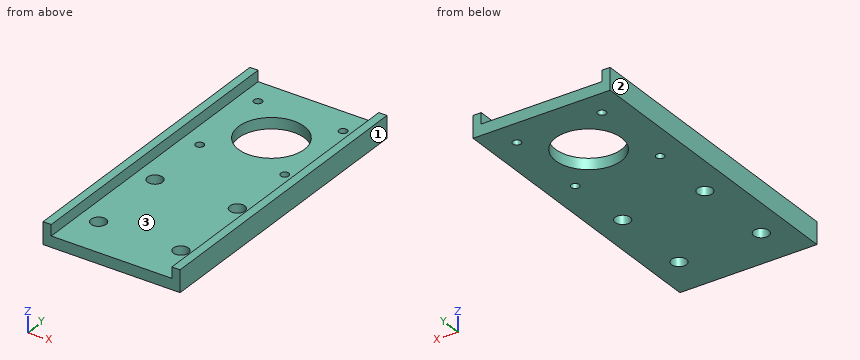
```python
from build123d import *

# Parameters (mm, degrees)
SKETCH1_W           = 50
SKETCH1_H           = 110
BOSS_EXTRUDE1_DEPTH = 4
CUT_EXTRUDE1_REACH  = 62.548
SKETCH2_R           = 1.5
CUT_EXTRUDE2_REACH  = 62.548
SKETCH3_R           = 2.75
SKETCH4_W           = 3
SKETCH4_H           = 110
BOSS_EXTRUDE2_DEPTH = 8
CUT_EXTRUDE3_REACH  = 62.943
SKETCH5_R           = 12


with BuildPart() as part:
    # Sketch1 → Boss-Extrude1 (new body)
    with BuildSketch(Plane.XY):
        Rectangle(SKETCH1_W, SKETCH1_H)
    extrude(amount=BOSS_EXTRUDE1_DEPTH)

    # Sketch2 → Cut-Extrude1 (cut, up to next)
    with BuildSketch(Plane.XY, mode=Mode.PRIVATE) as cut_extrude1_sk1:
        with Locations((-15.5, 45.5)):
            Circle(SKETCH2_R)
    cut_extrude1_tool1 = extrude(cut_extrude1_sk1.sketch, amount=CUT_EXTRUDE1_REACH, mode=Mode.PRIVATE) & part.part
    # Sketch2 → Cut-Extrude1 (cut, up to next)
    with BuildSketch(Plane.XY, mode=Mode.PRIVATE) as cut_extrude1_sk2:
        with Locations((-15.5, 14.5)):
            Circle(SKETCH2_R)
    cut_extrude1_tool2 = extrude(cut_extrude1_sk2.sketch, amount=CUT_EXTRUDE1_REACH, mode=Mode.PRIVATE) & part.part
    # Sketch2 → Cut-Extrude1 (cut, up to next)
    with BuildSketch(Plane.XY, mode=Mode.PRIVATE) as cut_extrude1_sk3:
        with Locations(Location((15.5, 14.5, 0), (0, 0, 180))):
            Circle(SKETCH2_R)
    cut_extrude1_tool3 = extrude(cut_extrude1_sk3.sketch, amount=CUT_EXTRUDE1_REACH, mode=Mode.PRIVATE) & part.part
    # Sketch2 → Cut-Extrude1 (cut, up to next)
    with BuildSketch(Plane.XY, mode=Mode.PRIVATE) as cut_extrude1_sk4:
        with Locations(Location((15.5, 45.5, 0), (0, 0, 180))):
            Circle(SKETCH2_R)
    cut_extrude1_tool4 = extrude(cut_extrude1_sk4.sketch, amount=CUT_EXTRUDE1_REACH, mode=Mode.PRIVATE) & part.part
    add(cut_extrude1_tool1.solids().sort_by_distance((-15.5, 45.5, 0))[0], mode=Mode.SUBTRACT)
    add(cut_extrude1_tool2.solids().sort_by_distance((-15.5, 14.5, 0))[0], mode=Mode.SUBTRACT)
    add(cut_extrude1_tool3.solids().sort_by_distance((15.5, 14.5, 0))[0], mode=Mode.SUBTRACT)
    add(cut_extrude1_tool4.solids().sort_by_distance((15.5, 45.5, 0))[0], mode=Mode.SUBTRACT)

    # Sketch3 → Cut-Extrude2 (cut, up to next)
    with BuildSketch(Plane.XY, mode=Mode.PRIVATE) as cut_extrude2_sk1:
        with Locations((-15, -40)):
            Circle(SKETCH3_R)
    cut_extrude2_tool1 = extrude(cut_extrude2_sk1.sketch, amount=CUT_EXTRUDE2_REACH, mode=Mode.PRIVATE) & part.part
    # Sketch3 → Cut-Extrude2 (cut, up to next)
    with BuildSketch(Plane.XY, mode=Mode.PRIVATE) as cut_extrude2_sk2:
        with Locations((-15, -10)):
            Circle(SKETCH3_R)
    cut_extrude2_tool2 = extrude(cut_extrude2_sk2.sketch, amount=CUT_EXTRUDE2_REACH, mode=Mode.PRIVATE) & part.part
    # Sketch3 → Cut-Extrude2 (cut, up to next)
    with BuildSketch(Plane.XY, mode=Mode.PRIVATE) as cut_extrude2_sk3:
        with Locations(Location((15, -40, 0), (0, 0, 180))):
            Circle(SKETCH3_R)
    cut_extrude2_tool3 = extrude(cut_extrude2_sk3.sketch, amount=CUT_EXTRUDE2_REACH, mode=Mode.PRIVATE) & part.part
    # Sketch3 → Cut-Extrude2 (cut, up to next)
    with BuildSketch(Plane.XY, mode=Mode.PRIVATE) as cut_extrude2_sk4:
        with Locations(Location((15, -10, 0), (0, 0, 180))):
            Circle(SKETCH3_R)
    cut_extrude2_tool4 = extrude(cut_extrude2_sk4.sketch, amount=CUT_EXTRUDE2_REACH, mode=Mode.PRIVATE) & part.part
    add(cut_extrude2_tool1.solids().sort_by_distance((-15, -40, 0))[0], mode=Mode.SUBTRACT)
    add(cut_extrude2_tool2.solids().sort_by_distance((-15, -10, 0))[0], mode=Mode.SUBTRACT)
    add(cut_extrude2_tool3.solids().sort_by_distance((15, -40, 0))[0], mode=Mode.SUBTRACT)
    add(cut_extrude2_tool4.solids().sort_by_distance((15, -10, 0))[0], mode=Mode.SUBTRACT)

    # Sketch4 → Boss-Extrude2 (add)
    with BuildSketch(Plane.XY):
        with Locations((-23.5, 0)):
            Rectangle(SKETCH4_W, SKETCH4_H)
        with Locations((23.5, 0)):
            Rectangle(SKETCH4_W, SKETCH4_H)
    extrude(amount=BOSS_EXTRUDE2_DEPTH)

    # Sketch5 → Cut-Extrude3 (cut, up to next)
    with BuildSketch(Plane.XY, mode=Mode.PRIVATE) as cut_extrude3_sk1:
        with Locations((0, 30)):
            Circle(SKETCH5_R)
    cut_extrude3_tool1 = extrude(cut_extrude3_sk1.sketch, amount=CUT_EXTRUDE3_REACH, mode=Mode.PRIVATE) & part.part
    add(cut_extrude3_tool1.solids().sort_by_distance((0, 30, 0))[0], mode=Mode.SUBTRACT)


solid = part.part
```
Design review of the part built by this model. Coordinates are the model's own, in mm. Face numbers are marked on the shaded views. Round coordinates to 2 decimals unless told otherwise and drop trailing zeros. Write each loop counter-clockwise with the first axis right and the second up, starting at its lowest first coordinate (ties: lowest second). Pieces come first, ordered by that corner, then holes. Notation, with made-up numbers: (25, -34) -> (58, -34) arc R30 ccw to (58, -1) -> close; hole circle Ø1 at (-24, 35). An arc over 180 degrees is marked (long way). Write item = value, one per line. Start each with the question number.
1) Wall thickness on probe 1 along X at (y, z) = (-10, 1.05); probe 2 along X at (y, z) = (45.5, 1.3); probe 3 along Y at (x, z) = (15.5, 1.1): over which ranges is each line inside the solid? List them lowest first. Write a range as from..to.
2) Take a section at D-D, the plane z = 1. Count the separate pieces of the cut face and the enclosed holes in it, plus the area to 3 significant figures.
3) Take a section at B-B, the plane z = 6.75. State the section outline as (x, y) points, plus the area to 3 significant figures.
4) Mouldability with a two-part tool opening along X and no side actions: class the marked faces 1, 2 and 3 as +X half, -X half, draft (parallel to the pull), parting line (faces both ways), or undercut.
5) Take a section at C-C, the plane y = 30. State the section outline as (x, z) points.
6) Take a section at A-A, the plane x = 0. State the section outline as (y, z) points.
7) Clearance check with a flat-ended pin moving along its axis: pin 1 (10 mm diameter, centred on x = 2.5, y = 39.5, fed in from +Z). State where the tip first meets the part, or that it passes through.
Results list:
q1.probe_1 = -25..-17.75, -12.25..12.25, 17.75..25
q1.probe_2 = -25..-17, -14..14, 17..25
q1.probe_3 = -55..-42.7, -37.3..-12.7, -7.3..13, 16..44, 47..55
q2.separate_pieces = 1
q2.enclosed_holes = 9
q2.area = 4,920 mm²
q3.outline = (-25, -55) -> (-22, -55) -> (-22, 55) -> (-25, 55) -> close; (22, -55) -> (25, -55) -> (25, 55) -> (22, 55) -> close
q3.area = 660 mm²
q4.face_1 = +X half
q4.face_2 = -X half
q4.face_3 = undercut
q5.outline = (-25, 0) -> (-12, 0) -> (-12, 4) -> (-22, 4) -> (-22, 8) -> (-25, 8) -> close; (12, 0) -> (25, 0) -> (25, 8) -> (22, 8) -> (22, 4) -> (12, 4) -> close
q6.outline = (-55, 0) -> (18, 0) -> (18, 4) -> (-55, 4) -> close; (42, 0) -> (55, 0) -> (55, 4) -> (42, 4) -> close
q7.pin_1 = 4
